```python
from build123d import *

# Parameters (mm, degrees)
SKETCH_1_W           = 44
SKETCH_1_H           = 34
EXTRUDE_1_DEPTH      = 24
CUT_EXTRUDE_1_DEPTH  = 31
SKETCH_5_W           = 23
SKETCH_5_H           = 10.5
EXTRUDE_4_DEPTH      = 1
EXTRUDE_5_DEPTH      = 23
SKETCH_7_R           = 1.8
CUT_EXTRUDE_2_DEPTH  = 23
CUT_EXTRUDE_4_DEPTH  = 19
CHAMFER_2_SIZE       = 2
CHAMFER_2_SIZE2      = 3
SKETCH_11_R          = 1.7
EXTRUDE_6_DEPTH      = 20
CUT_EXTRUDE_7_DEPTH  = 4
CHAMFER_3_SIZE       = 2.4
SKETCH_14_W          = 40.8
SKETCH_14_H          = 4
CUT_EXTRUDE_8_DEPTH  = 18
SKETCH_15_W          = 44
SKETCH_15_H          = 1
CUT_EXTRUDE_9_DEPTH  = 24
SKETCH_16_W          = 3.2
SKETCH_16_H          = 13.6
CUT_EXTRUDE_10_DEPTH = 5
SKETCH_17_W          = 1.6
SKETCH_17_H          = 4
CUT_EXTRUDE_11_DEPTH = 7.4
CUT_EXTRUDE_12_DEPTH = 7
SKETCH_19_W          = 1
SKETCH_19_H          = 10.5
CUT_EXTRUDE_13_DEPTH = 23
CHAMFER_4_SIZE       = 1.5
CHAMFER_5_SIZE       = 3
CHAMFER_5_SIZE2      = 2


with BuildPart() as part:
    # Sketch 1 → Extrude 1 (new body)
    with BuildSketch(Plane.XY):
        with Locations((0, 27)):
            Rectangle(SKETCH_1_W, SKETCH_1_H)
    extrude(amount=EXTRUDE_1_DEPTH)

    # Sketch 2 → Cut-Extrude 1 (cut)
    with BuildSketch(Plane(origin=(0, 44, 0), x_dir=(1, 0, 0), z_dir=(0, 1, 0))):
        Polygon((-18.8, 0), (18.8, 0), (18.8, -20), (20.4, -20), (20.4, -22), (18.8, -22), (18.8, -24), (-18.8, -24), (-18.8, -22), (-20.4, -22), (-20.4, -20), (-18.8, -20), align=None)
    extrude(amount=-CUT_EXTRUDE_1_DEPTH, mode=Mode.SUBTRACT)



with BuildPart() as body_2:
    # Sketch 5 → Extrude 4 (new body)
    with BuildSketch(Plane(origin=(0, 0, 0), x_dir=(-1, 0, 0), z_dir=(0, 0, -1))):
        with Locations((0, 4.75)):
            Rectangle(SKETCH_5_W, SKETCH_5_H)
    extrude(amount=EXTRUDE_4_DEPTH)


with BuildPart() as part_1:
    add(part.part)

    add(body_2.part)  # Extrude 5 merges body 2
    # Sketch 6 → Extrude 5 (add)
    with BuildSketch(Plane(origin=(11.5, 0, 0), x_dir=(0, 0, -1), z_dir=(1, 0, 0))):
        Polygon((0, -0.5), (-7, -0.5), (-24, 10), (0, 10), align=None)
    extrude(amount=-EXTRUDE_5_DEPTH)

    # Sketch 7 → Cut-Extrude 2 (cut)
    with BuildSketch(Plane.ZY.offset(11.5)):
        with Locations(Location((3, 3.5, 0), (0, 0, 270))):
            Circle(SKETCH_7_R)
    extrude(amount=-CUT_EXTRUDE_2_DEPTH, mode=Mode.SUBTRACT)

    # Sketch 8 → Cut-Extrude 4 (cut)
    with BuildSketch(Plane.ZY.offset(9.5)):
        Polygon((0, 8), (20, 13), (0, 13), align=None)
    extrude(amount=-CUT_EXTRUDE_4_DEPTH, mode=Mode.SUBTRACT)

    # Chamfer 2
    chamfer_2_edges = [part_1.edges().sort_by_distance(p)[0] for p in [
        (9.5, 13, 10),
    ]]
    chamfer_2_side = [part_1.faces().sort_by_distance(p)[0] for p in [
        (-18.32664601, 13, 10),
    ]]
    chamfer(chamfer_2_edges, length=CHAMFER_2_SIZE, length2=CHAMFER_2_SIZE2, reference=chamfer_2_side[0])

    # Sketch 11 → Extrude 6 (add)
    # profile 1 of 2: a face of its own
    with BuildSketch(Plane(origin=(0, 0, 0), x_dir=(-1, 0, 0), z_dir=(0, 0, -1))):
        with BuildLine():
            Line((-14, 43), (-18.8, 43))
            Line((-18.8, 43), (-18.8, 35.6))
            Line((-18.8, 35.6), (-14, 35.6))
            ThreePointArc((-14, 35.6), (-10.3, 39.3), (-14, 43))
        make_face()
        with Locations((-14, 39.3)):
            Circle(SKETCH_11_R, mode=Mode.SUBTRACT)
    # profile 2 of 2: a face of its own
    with BuildSketch(Plane(origin=(0, 0, 0), x_dir=(-1, 0, 0), z_dir=(0, 0, -1))):
        with BuildLine():
            Line((18.8, 35.6), (14, 35.6))
            ThreePointArc((14, 35.6), (10.3, 39.3), (14, 43))
            Line((14, 43), (18.8, 43))
            Line((18.8, 43), (18.8, 35.6))
        make_face()
        with Locations((14, 39.3)):
            Circle(SKETCH_11_R, mode=Mode.SUBTRACT)
    extrude(amount=-EXTRUDE_6_DEPTH)

    # Sketch 13 → Cut-Extrude 7 (cut)
    with BuildSketch(Plane.ZY.offset(22)):
        Polygon((9, 34), (17, 36), (17, 33.5), (9, 31.5), align=None)
        Polygon((9, 30.5), (17, 32.5), (17, 30), (9, 28), align=None)
        Polygon((9, 27), (17, 29), (17, 26.5), (9, 24.5), align=None)
        Polygon((9, 23.5), (17, 25.5), (17, 23), (9, 21), align=None)
        Polygon((9, 20), (17, 22), (17, 19.5), (9, 17.5), align=None)
    cut_extrude_7 = extrude(amount=-CUT_EXTRUDE_7_DEPTH, mode=Mode.SUBTRACT)

    # Mirror 1: Cut-Extrude 7 across plane
    add(cut_extrude_7.mirror(Plane(origin=(0, 0, 0), x_dir=(0, 0, 1), z_dir=(1, 0, 0))), mode=Mode.SUBTRACT)

    # Chamfer 3
    chamfer_3_edges = [part_1.edges().sort_by_distance(p)[0] for p in [
        (22, 10, 12),
        (-22, 10, 12),
    ]]
    chamfer(chamfer_3_edges, length=CHAMFER_3_SIZE)

    # Sketch 14 → Cut-Extrude 8 (cut)
    with BuildSketch(Plane(origin=(0, 44, 0), x_dir=(1, 0, 0), z_dir=(0, 1, 0))):
        with Locations((0, -22)):
            Rectangle(SKETCH_14_W, SKETCH_14_H)
    extrude(amount=-CUT_EXTRUDE_8_DEPTH, mode=Mode.SUBTRACT)

    # Sketch 15 → Cut-Extrude 9 (cut)
    with BuildSketch(Plane(origin=(0, 0, 0), x_dir=(-1, 0, 0), z_dir=(0, 0, -1))):
        with Locations((0, 43.5)):
            Rectangle(SKETCH_15_W, SKETCH_15_H)
    extrude(amount=-CUT_EXTRUDE_9_DEPTH, mode=Mode.SUBTRACT)

    # Sketch 16 → Cut-Extrude 10 (cut)
    with BuildSketch(Plane.XY.offset(24)):
        with Locations((20.4, 28.8)):
            Rectangle(SKETCH_16_W, SKETCH_16_H)
    extrude(amount=-CUT_EXTRUDE_10_DEPTH, mode=Mode.SUBTRACT)

    # Sketch 17 → Cut-Extrude 11 (cut)
    with BuildSketch(Plane(origin=(0, 43, 0), x_dir=(1, 0, 0), z_dir=(0, 1, 0))):
        with Locations((21.2, -22)):
            Rectangle(SKETCH_17_W, SKETCH_17_H)
    extrude(amount=-CUT_EXTRUDE_11_DEPTH, mode=Mode.SUBTRACT)

    # Sketch 18 → Cut-Extrude 12 (cut)
    with BuildSketch(Plane(origin=(0, 0, 0), x_dir=(-1, 0, 0), z_dir=(0, 0, -1))):
        Polygon((-22, 43), (-17, 43), (-17, 10), (-19.6, 10), (-22, 12.4), align=None)
        Polygon((22, 12.4), (19.6, 10), (17, 10), (17, 43), (22, 43), align=None)
    extrude(amount=-CUT_EXTRUDE_12_DEPTH, mode=Mode.SUBTRACT)

    # Sketch 19 → Cut-Extrude 13 (cut)
    with BuildSketch(Plane.ZY.offset(11.5)):
        with Locations((-0.5, 4.75)):
            Rectangle(SKETCH_19_W, SKETCH_19_H)
    extrude(amount=-CUT_EXTRUDE_13_DEPTH, mode=Mode.SUBTRACT)

    # Chamfer 4
    chamfer_4_edges = [part_1.edges().sort_by_distance(p)[0] for p in [
        (0, -0.5, 0),
    ]]
    chamfer(chamfer_4_edges, length=CHAMFER_4_SIZE)

    # Chamfer 5
    chamfer_5_edges = [part_1.edges().sort_by_distance(p)[0] for p in [
        (-9.5, 13, 10),
    ]]
    chamfer_5_side = [part_1.faces().sort_by_distance(p)[0] for p in [
        (-9.5, 11.333333333, 6.666666667),
    ]]
    chamfer(chamfer_5_edges, length=CHAMFER_5_SIZE, length2=CHAMFER_5_SIZE2, reference=chamfer_5_side[0])


solid = part_1.part
```
Work out the finished part from the listing and answer in its coordinate system (mm). A direction names the side the tool comes from. Coordinates: 2 decimals unless noted, no trailing zeros. Order: outer loops, then holes, each group sorted by start corner. A loop starts at its lowest first (then second) coordinate and runs counter-clockwise, first axis right, second up. Notation, with made-up numbers: (-16, 34.25) - (-5, 34.25) arc R14 ccw to (-5, 40.25) - close; hole circle Ø5 at (41, 68). An arc over 180 degrees is marked (long way). Answer as a JSON object with one key per item and string values.
1. Consider line 1 (Y direction, x = -14, z = 14); line 2 (X direction, y = 13.5, z = 17.5); line 3 (Y direction, x = -17.5, z = 17.5). Determine where each line is inside the solid, lowest interval first.
Output values:
{"line 1": "y = 10 to 13, 35.6 to 37.6, 41 to 43", "line 2": "x = -22 to -18.8, 18.8 to 22", "line 3": "y = 10 to 13, 35.6 to 43"}
2. Find section B-B on y = 39.3. Determine the outline of the cut face in (x, z), plus the area to 3 significant figures.
Output values:
{"outline": "(-22, 7) - (-17, 7) - (-17, 0) - (-15.7, 0) - (-15.7, 20) - (-20.4, 20) - (-20.4, 24) - (-22, 24) - close; (-12.3, 0) - (-10.3, 0) - (-10.3, 20) - (-12.3, 20) - close; (10.3, 0) - (12.3, 0) - (12.3, 20) - (10.3, 20) - close; (15.7, 0) - (17, 0) - (17, 7) - (22, 7) - (22, 20) - (15.7, 20) - close", "area": "268 mm²"}
3. Find section C-C on x = -1. Determine the outline of the cut face in (y, z).
Output values:
{"outline": "(-0.5, 1.5) - (1, 0) - (8, 0) - (13, 20) - (13, 24) - (10, 24) - (-0.5, 7) - close; hole circle Ø3.6 at (3.5, 3)"}
4. The mould has two halves that part along Z. Classify faces 6 (the face through (-20, 19, 9)), 7 (the face through (16, 39, 20)), 8 (the face through (12, 39, 0)), 9 (the face through (17, 12, 3)): +Z half, -Z half, draft (parallel to the pull), parting line (faces both ways), or undercut.
Output values:
{"face 6": "undercut", "face 7": "+Z half", "face 8": "-Z half", "face 9": "draft"}
5. Find section A-A on z = 3. Determine the outline of the cut face in (x, y), plus the area to 3 significant figures.
Output values:
{"outline": "(-17, 10) - (-11.5, 10) - (-11.5, 5.3) - (11.5, 5.3) - (11.5, 10) - (17, 10) - (17, 13) - (11.5, 13) - (9.5, 10) - (9.5, 8.75) - (-9.5, 8.75) - (-9.5, 10) - (-11.5, 13) - (-17, 13) - close; (-17, 35.6) - (-14, 35.6) arc R3.7 ccw to (-14, 43) - (-17, 43) - close; (-11.5, -0.5) - (11.5, -0.5) - (11.5, 1.7) - (-11.5, 1.7) - close; (14, 35.6) - (17, 35.6) - (17, 43) - (14, 43) arc R3.7 ccw to start; hole circle Ø3.4 at (-14, 39.3); hole circle Ø3.4 at (14, 39.3)", "area": "243 mm²"}
6. Each of these flat-tipped pins is pushed along its axis until it touches: P1, Ø2, axis at y = 4, z = 9, coming from the -X side; P2, Ø0.8, axis at x = 19.5, y = 29, coming from the +Z side; P3, Ø1.2, axis at x = -20, y = 25, coming from the -Z side. Where does it stop, or does it pass through?
Output values:
{"P1": "stops at x = -11.5", "P2": "stops at z = 19", "P3": "stops at z = 7"}
7. A tool of negligible diameter and unlimited length cuts with its end or side. For faces 1 (the face through (-20, 28, 13)), 2 (the face through (-16, 35.6, 10)), 3 (the face through (-17, 36, 20)), 4 (the face through (10.7, 11.8, 7.9)), 5 (the face through (20, 27, 7)), from which of +Z, -Z, +X, -X, +Y, -Y can it reach the whole face along a straight path? Write none if from no direction.
Output values:
{"face 1": "+X, -X", "face 2": "+Z, -Z", "face 3": "+Y", "face 4": "-Z", "face 5": "-Z, +X, +Y, -Y"}
8. Find section D-D on y = 16. Determine the outline of the cut face in (x, z).
Output values:
{"outline": "(-22, 7) - (-18.8, 7) - (-18.8, 20) - (-20.4, 20) - (-20.4, 22) - (-18.8, 22) - (-18.8, 24) - (-22, 24) - close; (18.8, 7) - (22, 7) - (22, 24) - (18.8, 24) - (18.8, 22) - (20.4, 22) - (20.4, 20) - (18.8, 20) - close"}
